The model under review builds one solid part; all positions refer to its coordinate system, in mm. A direction names the side the tool comes from. Round coordinates to 2 decimals unless told otherwise and drop trailing zeros. Order: outer loops, then holes, each group sorted by start corner. A loop starts at its lowest first (then second) coordinate and runs counter-clockwise, first axis right, second up.
1) Mouldability with a two-part tool opening along Y and no side actions: class faces 1 (the face through (127.09, 26.91, 20.53)), 2 (the face through (128, 21, 11)), 3 (the face through (73, 4, 5)), 4 (the face through (38, 23, 20)) as pulls with the +Y half, pulls with the -Y half, needs draft (parallel to the pull), parting line crosses it, or undercut.
2) Consider section B-B (x = 73). Give the boundary of the cut face in (y, z), then the cut area to 3 significant figures.
3) Consider section A-A (x = 24). Give the boundary of the cut face in (y, z), then the cut area to 3 significant figures.
4) To check wall thickness, follow L1, parallel to Y at x = 21, z = 39.1; L2, parallel to Z at x = 30, y = 17; L3, parallel to Z at x = 91.5, y = 27. State the ranges of each line that lie inside material, in increasing order.
5) Consider section D-D (x = 144.5). Give the boundary of the cut face in (y, z).
6) Machinability: for faces 5 (the face through (106.26, 3.13, 16.86)), 6 (the face through (70.71, 3.021, 17.965)), 7 (the face through (92.278, 2.618, 6.676)), 8 (the face through (37.93, 8.43, 12)), 9 (the face through (111.24, 26.98, 16.14)), which of the approach directions +Z, -Z, +X, -X, +Y, -Y give a long, thin tool a straight path to every point of the face, cutting with its end or side? Answer none if there is none.
7) Consider section C-C (y = 9). Give the number of separate pieces and of enclosed holes in the cut face, then the cut area to 3 significant figures.
8) Clearance check with flat-ended pins moving along their axes: P1, Ø19, axis at x = 100, z = 11, coming from the +Y side; P2, Ø14.5, axis at y = 18.5, z = 30, coming from the +X side; P3, Ø3, axis at x = 135.5, z = 21.5, coming from the -Y side; P4, Ø13.5, axis at x = 21, y = 15, coming from the -Z side. State where each tip first meets the part, or that it passes through.
from build123d import *
from build123d.topology import SkipClean

# Parameters (mm, degrees)
ESQUISSE1_W                   = 150
ESQUISSE1_H                   = 30
BOSS_EXTRU_1_DEPTH            = 40.5
BOSS_EXTRU_2_DEPTH            = 40.5
ENL_V_MAT_EXTRU_2_DEPTH       = 173.526084984
ENL_V_START                   = -138
ESQUISSE4_W                   = 31.5
ESQUISSE4_H                   = 44.902895409
ENL_V_MAT_EXTRU_3_DEPTH       = 50
ENL_V_START_2                 = -50
ENL_V_MAT_EXTRU_4_DEPTH       = 50
ESQUISSE6_W                   = 40.808644438
ESQUISSE6_H                   = 31.212282358
ENL_V_MAT_EXTRU_5_DEPTH       = 0.5
ESQUISSE7_W                   = 30.686861219
ESQUISSE7_H                   = 47.66257168
ENL_V_MAT_EXTRU_6_DEPTH       = 0.5
ENL_V_MAT_EXTRU_7_DEPTH       = 168.750558866
CONG_1_R                      = 2
CONG_2_R                      = 10
ESQUISSE9_W                   = 19.5
ESQUISSE9_H                   = 16
ENL_V_MAT_EXTRU_8_DEPTH       = 147.915792208
ENL_V_MAT_EXTRU_9_DEPTH       = 169.654641001
CONG_4_R                      = 5
ENL_V_MAT_EXTRU_10_DEPTH      = 168.750558866
ENL_V_MAT_EXTRU_10_DEPTH_BACK = 168.750558866
ENL_V_MAT_EXTRU_11_DEPTH      = 168.750558866
ESQUISSE13_R                  = 7.5
ENL_V_MAT_EXTRU_12_DEPTH      = 168.750558908
ENL_V_MAT_EXTRU_13_DEPTH      = 168.750558908
ENL_V_START_3                 = -105
ESQUISSE15_W                  = 31.5
ESQUISSE15_H                  = 62.544521206
ENL_V_MAT_EXTRU_14_DEPTH      = 45
CONG_5_R                      = 2
CONG_6_R                      = 5


with BuildPart() as part:
    # Esquisse1 → Boss.-Extru.1 (new body)
    with BuildSketch(Plane.XY):
        with Locations((75, 15)):
            Rectangle(ESQUISSE1_W, ESQUISSE1_H)
    extrude(amount=BOSS_EXTRU_1_DEPTH)

    # Esquisse3 → Boss.-Extru.2 (add, through all)
    with BuildSketch(Plane.XY.offset(40.5)):
        with BuildLine():
            Line((150, 7.5), (150, 0))
            ThreePointArc((150, 0), (165, 15), (150, 30))
            Line((150, 30), (150, 22.5))
            ThreePointArc((150, 22.5), (155.303300859, 20.303300859), (157.5, 15))
            ThreePointArc((157.5, 15), (155.303300859, 9.696699141), (150, 7.5))
        make_face()
    extrude(amount=-BOSS_EXTRU_2_DEPTH)

    # Esquisse3<3> → Enlèv. mat.-Extru.2 (cut, through all)
    with SkipClean():  # the faces are left unmerged after this step: merging them gives an invalid solid
        with BuildSketch(Plane.XY.offset(40.5)):
            with BuildLine():
                Line((150, 22.5), (150, 7.5))
                ThreePointArc((150, 7.5), (155.303300859, 9.696699141), (157.5, 15))
                ThreePointArc((157.5, 15), (155.303300859, 20.303300859), (150, 22.5))
            make_face()
            with BuildLine():
                ThreePointArc((150, 22.5), (142.5, 15), (150, 7.5))
                Line((150, 7.5), (150, 22.5))
            make_face()
        extrude(amount=-ENL_V_MAT_EXTRU_2_DEPTH, mode=Mode.SUBTRACT)

    # Esquisse4 → Enlèv. mat.-Extru.3 (cut)
    with BuildSketch(Plane.ZY.offset(ENL_V_START)):
        with Locations((20.25, 16.046124804)):
            Rectangle(ESQUISSE4_W, ESQUISSE4_H)
    extrude(amount=-ENL_V_MAT_EXTRU_3_DEPTH, mode=Mode.SUBTRACT)

    # Esquisse5 → Enlèv. mat.-Extru.4 (cut)
    with BuildSketch(Plane(origin=(0, 0, 0), x_dir=(-1, 0, 0), z_dir=(0, 0, -1)).offset(ENL_V_START_2)):
        with BuildLine():
            Line((-90, 0), (-150, 5))
            ThreePointArc((-150, 5), (-160, 15), (-150, 25))
            Line((-150, 25), (-90, 30))
            Line((-90, 30), (-150, 30))
            ThreePointArc((-150, 30), (-165, 15), (-150, 0))
            Line((-150, 0), (-90, 0))
        make_face()
    extrude(amount=ENL_V_MAT_EXTRU_4_DEPTH, mode=Mode.SUBTRACT)

    # Esquisse6 → Enlèv. mat.-Extru.5 (cut)
    with BuildSketch(Plane(origin=(0, 0, 0), x_dir=(-1, 0, 0), z_dir=(0, 0, -1))):
        with Locations((-159.466318707, 17.991552194)):
            Rectangle(ESQUISSE6_W, ESQUISSE6_H)
    extrude(amount=-ENL_V_MAT_EXTRU_5_DEPTH, mode=Mode.SUBTRACT)

    # Esquisse7 → Enlèv. mat.-Extru.6 (cut)
    with BuildSketch(Plane.XY.offset(40.5)):
        with Locations((150.623308265, 11.626621639)):
            Rectangle(ESQUISSE7_W, ESQUISSE7_H)
    extrude(amount=-ENL_V_MAT_EXTRU_6_DEPTH, mode=Mode.SUBTRACT)

    # Esquisse8 → Enlèv. mat.-Extru.7 (cut, through all)
    with BuildSketch(Plane(origin=(0, 0, 0), x_dir=(-1, 0, 0), z_dir=(0, 0, -1))):
        with BuildLine():
            Line((-127, 5), (-89, 5))
            ThreePointArc((-89, 5), (-88.292893219, 5.292893219), (-88, 6))
            Line((-88, 6), (-88, 24))
            ThreePointArc((-88, 24), (-88.292893219, 24.707106781), (-89, 25))
            Line((-89, 25), (-127, 25))
            ThreePointArc((-127, 25), (-127.707106781, 24.707106781), (-128, 24))
            Line((-128, 24), (-128, 6))
            ThreePointArc((-128, 6), (-127.707106781, 5.292893219), (-127, 5))
        make_face()
    extrude(amount=-ENL_V_MAT_EXTRU_7_DEPTH, mode=Mode.SUBTRACT)

    # Congé1
    cong_1_edges = [part.edges().sort_by_distance(p)[0] for p in [
        (138, 15, 36),
        (138, 15, 4.5),
    ]]
    fillet(cong_1_edges, radius=CONG_1_R)

    # Congé2
    # the kernel refuses this fillet: 10 mm, written as the material it takes off along each edge
    with BuildSketch(Plane(origin=(139.061996488, -3.717747791, 0), x_dir=(-1, 0, 0), z_dir=(0, 1, 0))) as cong_2_piece_1:
        with BuildLine():
            CenterArc((3.122498999, 10), CONG_2_R, 251.805127661, 18.194872339)
            Line((0, 0.5), (-0.06244998, 0.31))
            ThreePointArc((-0.06244998, 0.31), (-0.2, 0.25), (-0.2, 0))
            Line((-0.2, 0), (0, -0.2))
            Line((0, -0.2), (3.122498999, -0.2))
            Line((3.122498999, -0.2), (3.122498999, 0))
        make_face()
    extrude(amount=37.435495581, mode=Mode.SUBTRACT)
    with BuildSketch(Plane(origin=(135.279877656, 34.03292436, 40.5), x_dir=(-2.2168933355567372e-12, 0, -1.0), z_dir=(0, -1, 0))) as cong_2_piece_2:
        with BuildLine():
            CenterArc((10, -3.122498999), CONG_2_R, 161.805127661, 18.194872339)
            Line((0, -3.122498999), (-0.2, -3.122498999))
            Line((-0.2, -3.122498999), (-0.2, 0))
            Line((-0.2, 0), (0, 0.2))
            ThreePointArc((0, 0.2), (0.25, 0.2), (0.31, 0.06244998))
            Line((0.31, 0.06244998), (0.5, 0))
        make_face()
    extrude(amount=38.06584872, mode=Mode.SUBTRACT)

    # Esquisse9 → Enlèv. mat.-Extru.8 (cut, through all)
    with BuildSketch(Plane(origin=(138, 0, 0), x_dir=(0, 0, -1), z_dir=(1, 0, 0))):
        with Locations((-20.25, 15)):
            Rectangle(ESQUISSE9_W, ESQUISSE9_H)
    extrude(amount=-ENL_V_MAT_EXTRU_8_DEPTH, mode=Mode.SUBTRACT)

    # Esquisse10 → Enlèv. mat.-Extru.9 (cut, through all)
    with BuildSketch(Plane(origin=(0.620689655, -7.448275862, 0), x_dir=(0.9965457582448797, 0.08304547985373982, 0), z_dir=(0.08304547985373982, -0.9965457582448797, 0))):
        with BuildLine():
            Line((121.973972493, 23.536442559), (103.973972493, 8.536442559))
            ThreePointArc((103.973972493, 8.536442559), (103.373798137, 6.319149472), (105.254341292, 5))
            Line((105.254341292, 5), (123.254341292, 5))
            ThreePointArc((123.254341292, 5), (124.668554855, 5.585786438), (125.254341292, 7))
            Line((125.254341292, 7), (125.254341292, 22))
            ThreePointArc((125.254341292, 22), (124.102652085, 23.811178842), (121.973972493, 23.536442559))
        make_face()
        with BuildLine():
            Line((124.276260675, 31.963557441), (94.276260675, 6.963557441))
            ThreePointArc((94.276260675, 6.963557441), (92.147581083, 6.688821158), (90.995891876, 8.5))
            Line((90.995891876, 8.5), (90.995891876, 33.5))
            ThreePointArc((90.995891876, 33.5), (91.581678313, 34.914213562), (92.995891876, 35.5))
            Line((92.995891876, 35.5), (122.995891876, 35.5))
            ThreePointArc((122.995891876, 35.5), (124.876435031, 34.180850528), (124.276260675, 31.963557441))
        make_face()
    extrude(amount=-ENL_V_MAT_EXTRU_9_DEPTH, mode=Mode.SUBTRACT)

    # Congé4
    cong_4_edges = [part.edges().sort_by_distance(p)[0] for p in [
        (133, 23, 10.5),
        (133, 7, 10.5),
        (133, 7, 30),
        (133, 23, 30),
    ]]
    fillet(cong_4_edges, radius=CONG_4_R)

    # Esquisse11 → Enlèv. mat.-Extru.10 (cut, two sides: drawn at the far end of the back side and taken through both)
    with BuildSketch(Plane(origin=(0, 0, 0), x_dir=(-1, 0, 0), z_dir=(0, 0, -1)).offset(-ENL_V_MAT_EXTRU_10_DEPTH_BACK)):
        with BuildLine():
            Line((-82, 5), (-44, 5))
            ThreePointArc((-44, 5), (-43.292893219, 5.292893219), (-43, 6))
            Line((-43, 6), (-43, 24))
            ThreePointArc((-43, 24), (-43.292893219, 24.707106781), (-44, 25))
            Line((-44, 25), (-82, 25))
            ThreePointArc((-82, 25), (-82.707106781, 24.707106781), (-83, 24))
            Line((-83, 24), (-83, 6))
            ThreePointArc((-83, 6), (-82.707106781, 5.292893219), (-82, 5))
        make_face()
    extrude(amount=ENL_V_MAT_EXTRU_10_DEPTH + ENL_V_MAT_EXTRU_10_DEPTH_BACK, mode=Mode.SUBTRACT)

    # Esquisse12 → Enlèv. mat.-Extru.11 (cut, through all)
    with BuildSketch(Plane.XZ):
        with BuildLine():
            Line((81.75012438, 27.165281701), (59.356069146, 8.503569006))
            ThreePointArc((59.356069146, 8.503569006), (58.761473804, 6.306887113), (60.624536078, 5))
            Line((60.624536078, 5), (83.018591312, 5))
            ThreePointArc((83.018591312, 5), (84.419658831, 5.580341169), (85, 6.981408688))
            Line((85, 6.981408688), (85, 25.643121383))
            ThreePointArc((85, 25.643121383), (83.859016499, 27.437464131), (81.75012438, 27.165281701))
        make_face()
        with BuildLine():
            Line((79.569697683, 31.85680085), (49.569697683, 6.85680085))
            ThreePointArc((49.569697683, 6.85680085), (47.441018091, 6.582064567), (46.289328883, 8.393243409))
            Line((46.289328883, 8.393243409), (46.289328883, 33.393243409))
            ThreePointArc((46.289328883, 33.393243409), (46.875115321, 34.807456972), (48.289328883, 35.393243409))
            Line((48.289328883, 35.393243409), (78.289328883, 35.393243409))
            ThreePointArc((78.289328883, 35.393243409), (80.169872039, 34.074093937), (79.569697683, 31.85680085))
        make_face()
    extrude(amount=-ENL_V_MAT_EXTRU_11_DEPTH, mode=Mode.SUBTRACT)

    # Esquisse13 → Enlèv. mat.-Extru.12 (cut, through all)
    with BuildSketch(Plane(origin=(0, 0, 0), x_dir=(-1, 0, 0), z_dir=(0, 0, -1))):
        with Locations((-21, 15)):
            Circle(ESQUISSE13_R)
    extrude(amount=-ENL_V_MAT_EXTRU_12_DEPTH, mode=Mode.SUBTRACT)

    # Esquisse14 → Enlèv. mat.-Extru.13 (cut, through all)
    with BuildSketch(Plane(origin=(0, 0, 0), x_dir=(-1, 0, 0), z_dir=(0, 0, -1))):
        with BuildLine():
            Line((-21, 5), (-81, 0))
            Line((-81, 0), (-81, -20.615224629))
            Line((-81, -20.615224629), (7.927190419, -20.615224629))
            Line((7.927190419, -20.615224629), (9.55194442, 56.956421391))
            Line((9.55194442, 56.956421391), (-81, 56.956421391))
            Line((-81, 56.956421391), (-81, 30))
            Line((-81, 30), (-21, 25))
            ThreePointArc((-21, 25), (-11, 15), (-21, 5))
        make_face()
    extrude(amount=-ENL_V_MAT_EXTRU_13_DEPTH, mode=Mode.SUBTRACT)

    # Esquisse15 → Enlèv. mat.-Extru.14 (cut)
    with BuildSketch(Plane(origin=(138, 0, 0), x_dir=(0, 0, -1), z_dir=(1, 0, 0)).offset(ENL_V_START_3)):
        with Locations((-20.25, 10.635611164)):
            Rectangle(ESQUISSE15_W, ESQUISSE15_H)
    extrude(amount=-ENL_V_MAT_EXTRU_14_DEPTH, mode=Mode.SUBTRACT)

    # Congé5
    cong_5_edges = [part.edges().sort_by_distance(p)[0] for p in [
        (33, 15, 4.5),
        (33, 15, 36),
    ]]
    fillet(cong_5_edges, radius=CONG_5_R)

    # Congé6
    cong_6_edges = [part.edges().sort_by_distance(p)[0] for p in [
        (38, 23, 30),
        (38, 23, 10.5),
        (38, 7, 10.5),
        (38, 7, 30),
    ]]
    fillet(cong_6_edges, radius=CONG_6_R)


solid = part.part
Answer below:
1. face 1: pulls with the +Y half
1. face 2: undercut
1. face 3: needs draft
1. face 4: undercut
2. outline: (0.67, 0) - (5, 0) - (5, 5) - (0.67, 5) - close; (0.67, 19.87) - (5, 19.87) - (5, 26.38) - (0.67, 26.38) - close; (0.67, 35.39) - (5, 35.39) - (5, 40.5) - (0.67, 40.5) - close; (25, 0) - (29.33, 0) - (29.33, 5) - (25, 5) - close; (25, 19.87) - (29.33, 19.87) - (29.33, 26.38) - (25, 26.38) - close; (25, 35.39) - (29.33, 35.39) - (29.33, 40.5) - (25, 40.5) - close
2. area: 144 mm2
3. outline: (4.75, 0) - (8.13, 0) - (8.13, 4.5) - (4.75, 4.5) - close; (4.75, 36) - (8.13, 36) - (8.13, 40.5) - (4.75, 40.5) - close; (21.87, 0) - (25.25, 0) - (25.25, 4.5) - (21.87, 4.5) - close; (21.87, 36) - (25.25, 36) - (25.25, 40.5) - (21.87, 40.5) - close
3. area: 60.8 mm2
4. L1: y = 5 to 7.5, 22.5 to 25
4. L2: z = 0 to 4.5, 36 to 40.5
4. L3: z = 0 to 6.55, 35.5 to 40.5
5. outline: (4.54, 0.5) - (9.9, 0.5) - (9.9, 4.5) - (4.54, 4.5) - close; (4.54, 36) - (9.9, 36) - (9.9, 40) - (4.54, 40) - close; (20.1, 0.5) - (25.46, 0.5) - (25.46, 4.5) - (20.1, 4.5) - close; (20.1, 36) - (25.46, 36) - (25.46, 40) - (20.1, 40) - close
6. face 5: -Y
6. face 6: +Y, -Y
6. face 7: none
6. face 8: +X, -X
6. face 9: +Y
7. separate pieces: 10
7. enclosed holes: 0
7. area: 743 mm2
8. P1: stops at y = 29.87
8. P2: stops at x = 160
8. P3: stops at y = 3.67
8. P4: passes through
